For this review, take the finished solid that the model builds, in its own axes (mm). Face numbers are marked on the shaded views. A direction names the side the tool comes from. Give positions to 0.01 mm unless a question says otherwise; leave off trailing zeros. Write each loop counter-clockwise with the first axis right and the second up, starting at its lowest first coordinate (ties: lowest second). Pieces come first, ordered by that corner, then holes. Notation, with made-up numbers: M 58,-20.5 L 104,-20.5 A20 ccw 104,-11.5 Z; hole C -14.75,35.5 d11. An arc over 180 degrees is marked long. Answer as a JSON object with one key per item and string values. Group by question number.
```python
from build123d import *

# Parameters (mm, degrees)
PAD002_DEPTH          = 30
POCKET024_DEPTH       = 23
POLARPATTERN_COUNT    = 4
PAD013_DEPTH          = 12
POLARPATTERN001_COUNT = 4
SKETCH039_R           = 31
PAD014_DEPTH          = 42
SKETCH040_R           = 22.5
PAD015_DEPTH          = 105
SKETCH041_R           = 13.5
POCKET025_DEPTH       = 77
SKETCH042_R           = 11.75
POCKET026_DEPTH       = 50
POCKET027_DEPTH       = 15
POLARPATTERN002_COUNT = 4


with BuildPart() as part:
    # Sketch005 → Pad002 (new body)
    with BuildSketch(Plane.XY):
        with BuildLine():
            Line((-81, 131), (81, 131))
            ThreePointArc((131, 81), (116.355339, 116.355339), (81, 131))
            Line((131, 81), (131, -81))
            ThreePointArc((81, -131), (116.355339, -116.355339), (131, -81))
            Line((81, -131), (-81, -131))
            ThreePointArc((-131, -81), (-116.355339, -116.355339), (-81, -131))
            Line((-131, -81), (-131, 81))
            ThreePointArc((-81, 131), (-116.355339, 116.355339), (-131, 81))
        make_face()
    extrude(amount=PAD002_DEPTH)

    # Sketch037 (on Face9 of Pad002) → Pocket024 (cut)
    with BuildSketch(Plane(origin=(0, 0, 0), x_dir=(1, 0, 0), z_dir=(0, 0, -1))):
        with BuildLine():
            Line((-81, 121), (-5, 121))
            Line((-5, 121), (-5, 5))
            Line((-5, 5), (-121, 5))
            Line((-121, 5), (-121, 81))
            ThreePointArc((-81, 121), (-109.284271, 109.284271), (-121, 81))
        make_face()
    pocket024 = extrude(amount=-POCKET024_DEPTH, mode=Mode.SUBTRACT)

    # PolarPattern: Pocket024 ×4 about axis
    polarpattern_axis = Axis((0, 0, 0), (0, 0, -1))
    for i in range(1, POLARPATTERN_COUNT):
        add(pocket024.rotate(polarpattern_axis, i * 360 / POLARPATTERN_COUNT), mode=Mode.SUBTRACT)

    # Sketch038 (on Face5 of PolarPattern) → Pad013 (join)
    with BuildSketch(Plane.XY.offset(29.9)):
        Polygon((-12.391874, 12.391877), (99.536252, 124.332785), (105.391106, 122.550873), (110, 120), (120, 110), (124.952294, 101.341048), (12.337305, -12.337366), align=None)
    pad013 = extrude(amount=-PAD013_DEPTH)

    # PolarPattern001: Pad013 ×4 about axis
    polarpattern001_axis = Axis((0, 0, 29.9), (0, 0, 1))
    for i in range(1, POLARPATTERN001_COUNT):
        add(pad013.rotate(polarpattern001_axis, i * 360 / POLARPATTERN001_COUNT))

    # Sketch039 (on Face5 of PolarPattern001) → Pad014 (join)
    with BuildSketch(Plane.XY.offset(29.9)):
        Circle(SKETCH039_R)
    extrude(amount=-PAD014_DEPTH)

    # Sketch040 (on Face5 of Pad014) → Pad015 (join)
    with BuildSketch(Plane.XY.offset(29.9)):
        Circle(SKETCH040_R)
    extrude(amount=-PAD015_DEPTH)

    # Sketch041 (on Face54 of Pad015) → Pocket025 (cut)
    with BuildSketch(Plane(origin=(0, 0, -75.1), x_dir=(1, 0, 0), z_dir=(0, 0, -1))):
        Circle(SKETCH041_R)
    extrude(amount=-POCKET025_DEPTH, mode=Mode.SUBTRACT)

    # Sketch042 (on Face5 of Pocket025) → Pocket026 (cut)
    with BuildSketch(Plane.XY.offset(30)):
        Circle(SKETCH042_R)
    extrude(amount=-POCKET026_DEPTH, mode=Mode.SUBTRACT)

    # Sketch043 (on Face5 of Pocket026) → Pocket027 (cut)
    with BuildSketch(Plane.XY.offset(30)):
        with BuildLine():
            ThreePointArc((29.696699, 40.303301), (29.696699, 29.696699), (40.303301, 29.696699))
            Line((40.303301, 29.696699), (92.629203, 82.022601))
            ThreePointArc((92.629203, 82.022601), (92.629203, 92.629203), (82.022601, 92.629203))
            Line((82.022601, 92.629203), (29.696699, 40.303301))
        make_face()
    pocket027 = extrude(amount=-POCKET027_DEPTH, mode=Mode.SUBTRACT)

    # PolarPattern002: Pocket027 ×4 about axis
    polarpattern002_axis = Axis((0, 0, 30), (0, 0, 1))
    for i in range(1, POLARPATTERN002_COUNT):
        add(pocket027.rotate(polarpattern002_axis, i * 360 / POLARPATTERN002_COUNT), mode=Mode.SUBTRACT)


with BuildPart() as part_1:
    # Body002 placement: moved
    add(part.part.moved(Location((0, 210, -105))))


solid = part_1.part
```
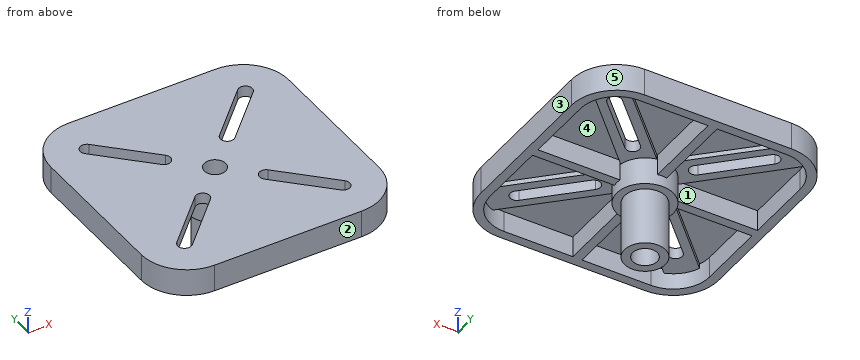
Item 1: Consider section B-B (x = 0). Give the boundary of the cut face in (y, z), plus the area to 3 significant figures.
Item 2: Insertion check: P1, Ø18.5, axis at x = 2.5, y = 219, coming from the -Z side; P2, Ø5, axis at x = 19, z = -163.5, coming from the +Y side. Each pin has a flat end and moves straight along its axis. Give the tip position at first contact, or say it passes through.
Item 3: Consider section C-C (z = -93.5). State how many separate pieces and enclosed holes the cut face has, plus the area to 3 significant figures.
Item 4: Consider section D-D (x = -35). Give the boundary of the cut face in (y, z), plus the area to 3 significant figures.
Item 5: To check wall thickness, follow probe 1 along Y at (x, z) = (-48, -99); probe 2 along X at (y, z) = (277, -92); probe 3 along Y at (x, z) = (0, -93). State the ranges of each line that lie inside material, in increasing order.
Item 6: Machinability: for the marked faces 4 and 5, which of the approach directions +Z, -Z, +X, -X, +Y, -Y give a long, thin tool a straight path to every point of the face, cutting with its end or side? Answer none if there is none.
Item 7: Draft analysis for pull direction Y (two halves, no side actions). For the marked faces 1, 2 and 3, state which applies: released by +Y, released by -Y, zero draft, split by the parting line, or undercut.
Item 8: Consider section A-A (y = 210). Give the boundary of the cut face in (x, z), plus the area to 3 significant figures.
Result set:
{
 "1": {"outline": "M 79,-105 L 179,-105 L 179,-117.1 L 187.5,-117.1 L 187.5,-180.1 L 196.5,-180.1 L 196.5,-103.1 L 198.25,-103.1 L 198.25,-75 L 79,-75 Z; M 221.75,-103.1 L 223.5,-103.1 L 223.5,-180.1 L 232.5,-180.1 L 232.5,-117.1 L 241,-117.1 L 241,-105 L 341,-105 L 341,-75 L 221.75,-75 Z", "area": "8,710 mm^2"},
 "2": {"P1": "stops at z = -180.1", "P2": "stops at y = 225.3"},
 "3": {"separate pieces": "1", "enclosed holes": "5", "area": "15,500 mm^2"},
 "4": {"outline": "M 79,-105 L 89,-105 L 89,-82 L 150.21,-82 L 150.21,-87.1 L 164.39,-87.1 L 164.39,-75 L 79,-75 Z; M 182.5,-87.1 L 199.46,-87.1 L 199.46,-82 L 205,-82 L 205,-105 L 215,-105 L 215,-82 L 220.21,-82 L 220.21,-87.1 L 237.5,-87.1 L 237.5,-75 L 182.5,-75 Z; M 255.61,-87.1 L 269.23,-87.1 L 269.23,-82 L 331,-82 L 331,-105 L 341,-105 L 341,-75 L 255.61,-75 Z", "area": "2,590 mm^2"},
 "5": {"probe 1": "y = 79 to 89, 205 to 215, 331 to 341", "probe 2": "x = -131 to -121, -5 to 5, 121 to 131", "probe 3": "y = 79 to 198.25, 221.75 to 341"},
 "6": {"face 4": "-Z", "face 5": "+Z, -Z, +X, +Y"},
 "7": {"face 1": "undercut", "face 2": "released by -Y", "face 3": "zero draft"},
 "8": {"outline": "M -131,-105 L -31,-105 L -31,-117.1 L -22.5,-117.1 L -22.5,-180.1 L -13.5,-180.1 L -13.5,-103.1 L -11.75,-103.1 L -11.75,-75 L -131,-75 Z; M 11.75,-103.1 L 13.5,-103.1 L 13.5,-180.1 L 22.5,-180.1 L 22.5,-117.1 L 31,-117.1 L 31,-105 L 131,-105 L 131,-75 L 11.75,-75 Z", "area": "8,710 mm^2"}
}
